Build history of the part. All positions in model axes, mm. Face numbers are marked on the shaded views. A direction names the side the tool comes from. Round coordinates to 2 decimals unless told otherwise and drop trailing zeros. Write each loop counter-clockwise with the first axis right and the second up, starting at its lowest first coordinate (ties: lowest second). Pieces come first, ordered by that corner, then holes. Notation, with made-up numbers: (56, 2.5) -> (109, 2.5) arc R23 ccw to (109, 30.5) -> close; hole circle Ø7 at (-4, -14). An arc over 180 degrees is marked (long way). Return JSON: item names as keys, results as strings.
from build123d import *

# Parameters (mm, degrees)
BOX_W           = 36
BOX_H           = 36
BOX_DEPTH       = 36
SKETCH002_R     = 3
POCKET_DEPTH    = 1
SKETCH_R        = 3
POCKET001_DEPTH = 1
SKETCH003_R     = 3
POCKET002_DEPTH = 1
SKETCH004_R     = 3
POCKET003_DEPTH = 1
SKETCH005_R     = 3
POCKET004_DEPTH = 1
SKETCH006_R     = 3
POCKET005_DEPTH = 1


with BuildPart() as sphere:
    # Sphere → Sphere (revolve)
    with BuildSketch(Plane.XZ):
        with BuildLine():
            ThreePointArc((0, -25), (25, 0), (0, 25))
            Line((0, 25), (0, -25))
        make_face()
    revolve(axis=Axis((0, 0, 0), (0, 0, 1)))


with BuildPart() as pocket005:
    # Box → Box (new body)
    with BuildSketch(Plane(origin=(-18, -18, -18), x_dir=(1, 0, 0), z_dir=(0, 0, 1))):
        with Locations((18, 18)):
            Rectangle(BOX_W, BOX_H)
    extrude(amount=BOX_DEPTH)

    # Common: intersect Sphere
    add(sphere.part, mode=Mode.INTERSECT)

    # Sketch002 → Pocket (cut)
    with BuildSketch(Plane.XY.offset(18)):
        with Locations((-8, 8)):
            Circle(SKETCH002_R)
        with Locations((-8, 0)):
            Circle(SKETCH002_R)
        with Locations((-8, -8)):
            Circle(SKETCH002_R)
        with Locations((8, 8)):
            Circle(SKETCH002_R)
        with Locations((8, -8)):
            Circle(SKETCH002_R)
        with Locations((8, 0)):
            Circle(SKETCH002_R)
    extrude(amount=-POCKET_DEPTH, mode=Mode.SUBTRACT)

    # Sketch → Pocket001 (cut)
    with BuildSketch(Plane.YZ.offset(18)):
        with Locations((-8, 8)):
            Circle(SKETCH_R)
        with Locations((8, 8)):
            Circle(SKETCH_R)
        with Locations((-7.883513, -8.046017)):
            Circle(SKETCH_R)
        with Locations((8, -8)):
            Circle(SKETCH_R)
        Circle(SKETCH_R)
    extrude(amount=-POCKET001_DEPTH, mode=Mode.SUBTRACT)

    # Sketch003 → Pocket002 (cut)
    with BuildSketch(Plane.XZ.offset(18)):
        with Locations((-8, 8)):
            Circle(SKETCH003_R)
        with Locations((8, 8)):
            Circle(SKETCH003_R)
        with Locations((8, -8)):
            Circle(SKETCH003_R)
        with Locations((-8, -8)):
            Circle(SKETCH003_R)
    extrude(amount=-POCKET002_DEPTH, mode=Mode.SUBTRACT)

    # Sketch004 → Pocket003 (cut)
    with BuildSketch(Plane(origin=(0, 18, 0), x_dir=(-1, 0, 0), z_dir=(0, 1, 0))):
        with Locations((-8, 8)):
            Circle(SKETCH004_R)
        Circle(SKETCH004_R)
        with Locations((8, -8)):
            Circle(SKETCH004_R)
    extrude(amount=-POCKET003_DEPTH, mode=Mode.SUBTRACT)

    # Sketch005 → Pocket004 (cut)
    with BuildSketch(Plane(origin=(0, 0, -18), x_dir=(1, 0, 0), z_dir=(0, 0, -1))):
        Circle(SKETCH005_R)
    extrude(amount=-POCKET004_DEPTH, mode=Mode.SUBTRACT)

    # Sketch006 → Pocket005 (cut)
    with BuildSketch(Plane(origin=(-18, 0, 0), x_dir=(0, -1, 0), z_dir=(-1, 0, 0))):
        with Locations((-8, 8)):
            Circle(SKETCH006_R)
        with Locations((8, -8)):
            Circle(SKETCH006_R)
    extrude(amount=-POCKET005_DEPTH, mode=Mode.SUBTRACT)


solid = pocket005.part
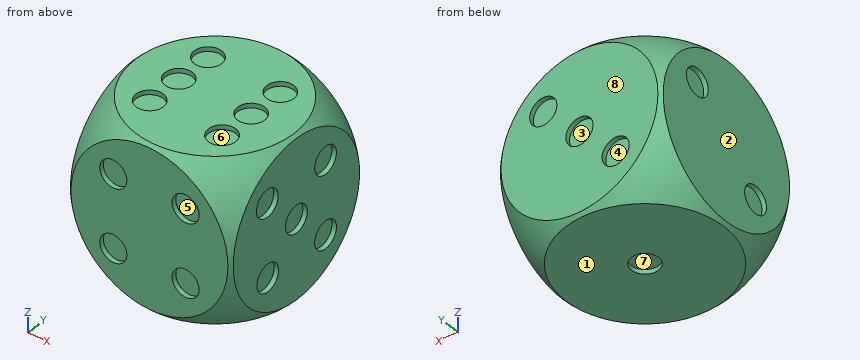
Q1. Wall check: L1, parallel to Z at x = -8, y = -17.15; L2, parallel to Z at x = 17.5, y = -8; L3, parallel to Z at x = 0, y = 17.65. Give the ranges that are in metal, low to high.
Verdict:
{"L1": "z = -16.34 to -11, -5 to 5, 11 to 16.34", "L2": "z = -15.96 to -11.04, -5.05 to 5, 11 to 15.96", "L3": "z = -17.71 to -3, 3 to 17.71"}
Q2. Pin check, flat tips, straight feed: pin 1 Ø3.5 at (x, z) = (-8, -8) entering from +Y; pin 2 Ø3 at (y, z) = (7.5, 9) entering from +X; pin 3 Ø1 at (x, z) = (10, 7.5) entering from -Y. Stop position of each tip, or through.
Verdict:
{"pin 1": "stops at y = 17", "pin 2": "stops at x = 17", "pin 3": "stops at y = -17"}
Q3. Saw through at A-A on y = 0. List the corners of the cut face in (x, z), then the cut area to 3 significant figures.
Verdict:
{"outline": "(-18, -17.35) arc R25 ccw to (-17.35, -18) -> (-3, -18) -> (-3, -17) -> (3, -17) -> (3, -18) -> (17.35, -18) arc R25 ccw to (18, -17.35) -> (18, -3) -> (17, -3) -> (17, 3) -> (18, 3) -> (18, 17.35) arc R25 ccw to (17.35, 18) -> (11, 18) -> (11, 17) -> (5, 17) -> (5, 18) -> (-5, 18) -> (-5, 17) -> (-11, 17) -> (-11, 18) -> (-17.35, 18) arc R25 ccw to (-18, 17.35) -> close", "area": "1,270 mm²"}
Q4. Two-plate mould, pull along Z, no slides. Class the marked faces 1, 2 and 3: +Z half, -Z half, draft (parallel to the pull), parting line (faces both ways), or undercut.
Verdict:
{"face 1": "-Z half", "face 2": "draft", "face 3": "undercut"}
Q5. 3-axis set-ups, long thin cutter, end or side, ignore diameter. For the marked faces 4, 5, 6, 7 and 8: which of +Z, -Z, +X, -X, +Y, -Y reach the whole face in a straight line?
Verdict:
{"face 4": "+Y", "face 5": "-Y", "face 6": "+Z", "face 7": "-Z", "face 8": "+Z, -Z, +X, -X, +Y"}
Q6. Saw through at D-D on y = -12. List the corners of the cut face in (x, z).
Verdict:
{"outline": "(-18, -12.53) arc R21.93 ccw to (-12.53, -18) -> (12.53, -18) arc R21.93 ccw to (18, -12.53) -> (18, 12.53) arc R21.93 ccw to (12.53, 18) -> (-12.53, 18) arc R21.93 ccw to (-18, 12.53) -> close"}
Q7. Saw through at C-C on y = 10. List the corners of the cut face in (x, z), then the cut area to 3 significant figures.
Verdict:
{"outline": "(-18, -14.18) arc R22.91 ccw to (-14.18, -18) -> (14.18, -18) arc R22.91 ccw to (18, -14.18) -> (18, -10.24) -> (17, -10.24) -> (17, -5.76) -> (18, -5.76) -> (18, 5.76) -> (17, 5.76) -> (17, 10.24) -> (18, 10.24) -> (18, 14.18) arc R22.91 ccw to (14.18, 18) -> (10.24, 18) -> (10.24, 17) -> (5.76, 17) -> (5.76, 18) -> (-5.76, 18) -> (-5.76, 17) -> (-10.24, 17) -> (-10.24, 18) -> (-14.18, 18) arc R22.91 ccw to (-18, 14.18) -> (-18, 10.24) -> (-17, 10.24) -> (-17, 5.76) -> (-18, 5.76) -> close", "area": "1,250 mm²"}
